```python
from build123d import *

# Parameters (mm, degrees)
SKETCH1_W           = 152.4
SKETCH1_H           = 52.832
BOSS_EXTRUDE1_DEPTH = 4.7625
SKETCH2_R           = 2.69
CUT_EXTRUDE1_DEPTH  = 81.789395729
SKETCH5_R           = 2.667
SKETCH5_R_2         = 2.54
CUT_EXTRUDE2_DEPTH  = 81.789395729
SKETCH6_W           = 52.832
SKETCH6_H           = 4.7625
BOSS_EXTRUDE2_DEPTH = 2
FILLET1_R           = 2.54


with BuildPart() as part:
    # Sketch1 → Boss-Extrude1 (new body)
    with BuildSketch(Plane(origin=(0, 0, 0), x_dir=(1, 0, 0), z_dir=(0, 1, 0))):
        Rectangle(SKETCH1_W, SKETCH1_H)
    extrude(amount=BOSS_EXTRUDE1_DEPTH)

    # Sketch2 → Cut-Extrude1 (cut, through all)
    with BuildSketch(Plane(origin=(0, 4.7625, 0), x_dir=(1, 0, 0), z_dir=(0, 1, 0))):
        with Locations(Location((68.607011479, -15.24, 0), (0, 0, 270))):
            Circle(SKETCH2_R)
        with Locations(Location((68.607011479, 0, 0), (0, 0, 270))):
            Circle(SKETCH2_R)
        with Locations(Location((68.607011479, 15.24, 0), (0, 0, 270))):
            Circle(SKETCH2_R)
    extrude(amount=-CUT_EXTRUDE1_DEPTH, mode=Mode.SUBTRACT)

    # Sketch5 → Cut-Extrude2 (cut, through all)
    with BuildSketch(Plane.XZ):
        with Locations(Location((-70.677366471, 15.3162, 0), (0, 0, 270))):
            Circle(SKETCH5_R)
        with Locations(Location((-70.677366471, 0.0762, 0), (0, 0, 270))):
            Circle(SKETCH5_R_2)
        with Locations(Location((-70.677366471, -15.1638, 0), (0, 0, 270))):
            Circle(SKETCH5_R_2)
    extrude(amount=-CUT_EXTRUDE2_DEPTH, mode=Mode.SUBTRACT)

    # Sketch6 → Boss-Extrude2 (add)
    with BuildSketch(Plane.ZY.offset(76.2)):
        with Locations((0, 2.38125)):
            Rectangle(SKETCH6_W, SKETCH6_H)
    extrude(amount=BOSS_EXTRUDE2_DEPTH)

    # Fillet1
    fillet1_edges = [part.edges().sort_by_distance(p)[0] for p in [
        (-78.2, 2.38125, 26.416),
        (-78.2, 2.38125, -26.416),
        (76.2, 2.38125, 26.416),
        (76.2, 2.38125, -26.416),
    ]]
    fillet(fillet1_edges, radius=FILLET1_R)


solid = part.part
```
Input: part model. Units: mm. Frame: model coordinates. Coordinates: 2 decimals unless noted, no trailing zeros. Loops run counter-clockwise (first coordinate to the right, second up) from the corner with the lowest first, then second, coordinate; pieces in that order, holes last.
Q1. Section B-B, the plane y = 3.2. Return the cut outline in (x, z).
Results are:
outline: (-78.2, -23.88) arc R2.54 ccw to (-75.66, -26.42) - (73.66, -26.42) arc R2.54 ccw to (76.2, -23.88) - (76.2, 23.88) arc R2.54 ccw to (73.66, 26.42) - (-75.66, 26.42) arc R2.54 ccw to (-78.2, 23.88) - close; hole circle Ø5.33 at (-70.68, 15.32); hole circle Ø5.08 at (-70.68, -15.16); hole circle Ø5.08 at (-70.68, 0.08); hole circle Ø5.38 at (68.61, -15.24); hole circle Ø5.38 at (68.61, 0); hole circle Ø5.38 at (68.61, 15.24)
Q2. Section C-C, the plane z = 0. Return the cut outline in (x, y), and give its area (3 significant figures).
Results are:
outline: (-78.2, 0) - (-73.22, 0) - (-73.22, 4.76) - (-78.2, 4.76) - close; (-68.14, 0) - (65.92, 0) - (65.92, 4.76) - (-68.14, 4.76) - close; (71.3, 0) - (76.2, 0) - (76.2, 4.76) - (71.3, 4.76) - close
area: 686 mm2
Q3. Mould query, pull axis X, two halves, no side actions, for faces 1 (the cylindrical face through (65.98, 2.41, -0.58)), 2 (the flat face through (0, 2, 26.416)), 3 (the cylindrical face through (-77.44, 2.41, -25.69)). Classes: +X half, -X half, draft (parallel to the pull), parting line (faces both ways), or undercut.
Results are:
face 1: undercut
face 2: draft
face 3: -X half
Q4. Line query: line 1 along X through (y, z) = (2.05, -15.24); line 2 along X through (y, z) = (4.25, -1); line 3 along Z through (x, y) = (68, 2.1). Output: solid intervals per line, ascending.
Results are:
line 1: x = -78.2 to -73.22, -68.14 to 65.92, 71.3 to 76.2
line 2: x = -78.2 to -72.98, -68.38 to 66.11, 71.1 to 76.2
line 3: z = -26.42 to -17.86, -12.62 to -2.62, 2.62 to 12.62, 17.86 to 26.42
Q5. Contact query for a flat-ended pin moving along its axis: pin 1 (4.5 mm diameter, centred on x = 68.61, z = 15.24, fed in from +Y). Output: stop coordinate, or through.
Results are:
pin 1: passes through
Q6. Section A-A, the plane z = 15.24. Return the cut outline in (x, y).
Results are:
outline: (-78.2, 0) - (-73.34, 0) - (-73.34, 4.76) - (-78.2, 4.76) - close; (-68.01, 0) - (65.92, 0) - (65.92, 4.76) - (-68.01, 4.76) - close; (71.3, 0) - (76.2, 0) - (76.2, 4.76) - (71.3, 4.76) - close
